from build123d import *

# Parameters (mm, degrees)
CROQUIS1_W              = 74
CROQUIS1_H              = 54
SALIENTE_EXTRUIR1_DEPTH = 6
CROQUIS3_W              = 9
CROQUIS3_H              = 5
SALIENTE_EXTRUIR2_DEPTH = 10
REDONDEO1_R             = 1
CORTAR_EXTRUIR1_DEPTH   = 100
CORTAR_EXTRUIR2_DEPTH   = 100
CORTAR_EXTRUIR3_DEPTH   = 70
CROQUIS8_W              = 8
CROQUIS8_H              = 6
CORTAR_EXTRUIR4_DEPTH   = 6
REDONDEO2_R             = 1
CROQUIS11_W             = 9
CROQUIS11_H             = 5
SALIENTE_EXTRUIR3_DEPTH = 5
REDONDEO3_R             = 1
CROQUIS17_R             = 1
CORTAR_EXTRUIR10_DEPTH  = 100
CROQUIS18_R             = 2
CORTAR_EXTRUIR11_DEPTH  = 1
CORTAR_EXTRUIR12_START  = -1
CROQUIS19_R             = 2
CORTAR_EXTRUIR12_DEPTH  = 1
CROQUIS12_R             = 1
CORTAR_EXTRUIR7_DEPTH   = 100
CROQUIS15_R             = 2
CORTAR_EXTRUIR8_DEPTH   = 1
CORTAR_EXTRUIR9_START   = -1
CROQUIS16_R             = 2
CORTAR_EXTRUIR9_DEPTH   = 1


with BuildPart() as part:
    # Croquis1 → Saliente-Extruir1 (new, symmetric)
    with BuildSketch(Plane(origin=(0, 0, 0), x_dir=(1, 0, 0), z_dir=(0, 1, 0))):
        Rectangle(CROQUIS1_W, CROQUIS1_H)
    extrude(amount=SALIENTE_EXTRUIR1_DEPTH, both=True)

    # Croquis3 → Saliente-Extruir2 (add, symmetric)
    with BuildSketch(Plane(origin=(0, 6, 0), x_dir=(1, 0, 0), z_dir=(0, 1, 0))):
        with Locations((0, -28.5)):
            Rectangle(CROQUIS3_W, CROQUIS3_H)
        with Locations((0, 28.5)):
            Rectangle(CROQUIS3_W, CROQUIS3_H)
    extrude(amount=SALIENTE_EXTRUIR2_DEPTH, both=True)

    # Redondeo1
    redondeo1_edges = [part.edges().sort_by_distance(p)[0] for p in [
        (4.5, 6, 31),
        (-4.5, 6, 31),
        (4.5, 6, -31),
        (-4.5, 6, -31),
    ]]
    fillet(redondeo1_edges, radius=REDONDEO1_R)

    # Croquis5 → Cortar-Extruir1 (cut)
    with BuildSketch(Plane(origin=(37, 0, 0), x_dir=(0, 0, -1), z_dir=(1, 0, 0))):
        with BuildLine():
            Line((-31, -1.820778385), (-31, -6))
            Line((-31, -6), (-18.642754783, -6))
            ThreePointArc((-18.642754783, -6), (-25.098766863, -4.730582529), (-31, -1.820778385))
        make_face()
        with BuildLine():
            Line((31, -1.820778385), (31, -6))
            Line((31, -6), (18.642754783, -6))
            ThreePointArc((18.642754783, -6), (25.098766863, -4.730582529), (31, -1.820778385))
        make_face()
    extrude(amount=-CORTAR_EXTRUIR1_DEPTH, mode=Mode.SUBTRACT)

    # Croquis6 → Cortar-Extruir2 (cut)
    with BuildSketch(Plane.ZY.offset(37)):
        with BuildLine():
            Line((-27, -1), (-27, -4))
            Line((-27, -4), (-31, -4))
            Line((-31, -4), (-33.432664366, -4))
            Line((-33.432664366, -4), (-33.432664366, 2.46409105))
            Line((-33.432664366, 2.46409105), (-31, 2.46409105))
            ThreePointArc((-31, 2.46409105), (-29.791283854, -0.181653154), (-27, -1))
        make_face()
        with BuildLine():
            Line((27, -1), (27, -4))
            Line((27, -4), (31, -4))
            Line((31, -4), (33.432664366, -4))
            Line((33.432664366, -4), (33.432664366, 2.46409105))
            Line((33.432664366, 2.46409105), (31, 2.46409105))
            ThreePointArc((31, 2.46409105), (29.791283854, -0.181653154), (27, -1))
        make_face()
    extrude(amount=-CORTAR_EXTRUIR2_DEPTH, mode=Mode.SUBTRACT)

    # Croquis7 → Cortar-Extruir3 (cut)
    with BuildSketch(Plane.ZY.offset(35)):
        with BuildLine():
            Line((-25, 6), (25, 6))
            Line((25, 6), (25, -2))
            ThreePointArc((25, -2), (21.888320303, -3.212786251), (18.642754783, -4))
            Line((18.642754783, -4), (-18.642754783, -4))
            ThreePointArc((-18.642754783, -4), (-21.888320303, -3.212786251), (-25, -2))
            Line((-25, -2), (-25, 6))
        make_face()
    extrude(amount=-CORTAR_EXTRUIR3_DEPTH, mode=Mode.SUBTRACT)

    # Croquis8 → Cortar-Extruir4 (cut)
    with BuildSketch(Plane.XZ.offset(6)):
        Polygon((-31.805445069, 16), (-28.194554931, 11.20818694), (-28.194554931, 13), (-21.194554931, 13), (-21.194554931, 19), (-28.194554931, 19), (-28.194554931, 20.79181306), align=None)
        Polygon((24.194554931, 13), (17.194554931, 13), (17.194554931, 19), (24.194554931, 19), (24.194554931, 20.79181306), (27.805445069, 16), (24.194554931, 11.20818694), align=None)
        with Locations((-2, 23)):
            Rectangle(CROQUIS8_W, CROQUIS8_H)
    extrude(amount=-CORTAR_EXTRUIR4_DEPTH, mode=Mode.SUBTRACT)

    # Redondeo2
    redondeo2_edges = [part.edges().sort_by_distance(p)[0] for p in [
        (-6, -4.802427791, 20),
        (2, -4.802427791, 20),
        (2, -2.203209257, 26),
        (-6, -2.203209257, 26),
    ]]
    fillet(redondeo2_edges, radius=REDONDEO2_R - 0.0001)  # a hair under: the kernel refuses the full size

    # Croquis11 → Saliente-Extruir3 (add, symmetric)
    with BuildSketch(Plane(origin=(0, 16, 0), x_dir=(1, 0, 0), z_dir=(0, 1, 0))):
        with Locations((0, -28.5)):
            Rectangle(CROQUIS11_W, CROQUIS11_H)
        with Locations((0, 28.5)):
            Rectangle(CROQUIS11_W, CROQUIS11_H)
    extrude(amount=SALIENTE_EXTRUIR3_DEPTH, both=True)

    # Redondeo3
    redondeo3_edges = [part.edges().sort_by_distance(p)[0] for p in [
        (-4.5, 16, -31),
        (4.5, 16, -31),
        (-4.5, 16, 31),
        (4.5, 16, 31),
    ]]
    fillet(redondeo3_edges, radius=REDONDEO3_R)

    # Croquis17 → Cortar-Extruir10 (cut)
    with BuildSketch(Plane.XY.offset(31)):
        with Locations((0, 18)):
            Circle(CROQUIS17_R)
    extrude(amount=-CORTAR_EXTRUIR10_DEPTH, mode=Mode.SUBTRACT)

    # Croquis18 → Cortar-Extruir11 (cut)
    with BuildSketch(Plane.XY.offset(31)):
        with Locations((0, 18)):
            Circle(CROQUIS18_R)
    extrude(amount=-CORTAR_EXTRUIR11_DEPTH, mode=Mode.SUBTRACT)

    # Croquis19 → Cortar-Extruir12 (cut)
    with BuildSketch(Plane(origin=(0, 0, -31), x_dir=(-1, 0, 0), z_dir=(0, 0, -1)).offset(CORTAR_EXTRUIR12_START)):
        with Locations(Location((0, 18, 0), (0, 0, 180))):
            Circle(CROQUIS19_R)
    extrude(amount=CORTAR_EXTRUIR12_DEPTH, mode=Mode.SUBTRACT)

    # Croquis12 → Cortar-Extruir7 (cut)
    with BuildSketch(Plane.XY.offset(31)):
        with Locations(Location((0, 18, 0), (0, 0, 180))):
            Circle(CROQUIS12_R)
    extrude(amount=-CORTAR_EXTRUIR7_DEPTH, mode=Mode.SUBTRACT)

    # Croquis15 → Cortar-Extruir8 (cut)
    with BuildSketch(Plane.XY.offset(31)):
        with Locations((0, 18)):
            Circle(CROQUIS15_R)
    extrude(amount=-CORTAR_EXTRUIR8_DEPTH, mode=Mode.SUBTRACT)

    # Croquis16 → Cortar-Extruir9 (cut)
    with BuildSketch(Plane(origin=(0, 0, -31), x_dir=(-1, 0, 0), z_dir=(0, 0, -1)).offset(CORTAR_EXTRUIR9_START)):
        with Locations(Location((0, 18, 0), (0, 0, 180))):
            Circle(CROQUIS16_R)
    extrude(amount=CORTAR_EXTRUIR9_DEPTH, mode=Mode.SUBTRACT)


solid = part.part
Source: CAD feature listing. Evaluate the final solid. Frame: model axes, mm. A direction names the side the tool comes from. Give positions to 0.01 mm unless a question says otherwise; leave off trailing zeros. Write each loop counter-clockwise with the first axis right and the second up, starting at its lowest first coordinate (ties: lowest second). Pieces come first, ordered by that corner, then holes. Notation, with made-up numbers: (18, 59.5) -> (63, 59.5) arc R32 cw to (63, 95.5) -> close; hole circle Ø5 at (-36.5, -5). An arc over 180 degrees is marked (long way). Return JSON: item names as keys, results as strings. Group by question number.
1. Mould query, pull axis Y, two halves, no side actions, for faces 5 (the face through (-25, -5, 19)), 6 (the face through (0.518, -5.376, -22.849)), 7 (the face through (-0.26, 16.017, -30.493)). Classes: +Y half, -Y half, draft (parallel to the pull), parting line (faces both ways), or undercut.
2. Pin query (flat end, axial travel): pin 1 Ø2 at (x, y) = (-1.5, -2.5) entering from -Z; pin 2 Ø18.5 at (x, z) = (-3, 7) entering from +Y; pin 3 Ø1.2 at (y, z) = (13.5, -27.5) entering from -X. Return the tip coordinate at first contact, or that it passes through.
3. Section B-B, the plane x = 22.5. Output: boundary loops of the cut face in (y, z).
4. Section C-C, the plane z = 23.5. Output: boundary loops of the cut face in (x, y), then the cut area to 3 significant figures.
5. Section D-D, the plane x = -15. Output: boundary loops of the cut face in (y, z), then the cut area to 3 significant figures.
6. Access query for faces 1 (the face through (1, 19, -30)), 2 (the face through (1, 17, 30)), 3 (the face through (0, 2, -25)), 4 (the face through (-21.195, -5, 16)). Directions: +Z, -Z, +X, -X, +Y, -Y. A direction counts if a zero-diameter tool reaches every point of the face in a straight line with its end or side. Return the directions, or none.
7. Material intervals for line 1 (Z direction, x = -12.5, y = -1.75); line 2 (X direction, y = 18, z = -26.8); line 3 (Y direction, x = 27.5, z = 0), sorted ascending. Write a range as from..to.
8. Section A-A, the plane y = 18. Output: boundary loops of the cut face in (x, z).
Determined:
{
 "1": {"face 5": "draft", "face 6": "-Y half", "face 7": "undercut"},
 "2": {"pin 1": "stops at z = -27", "pin 2": "stops at y = -4", "pin 3": "stops at x = -4.5"},
 "3": {"outline": "(-6, -18.64) arc R25 ccw to (-4, -27) -> (6, -27) -> (6, -25) -> (-2, -25) arc R25 cw to (-4, -18.64) -> (-4, 13) -> (-6, 13) -> close; (-5.98, 19) -> (-3.94, 19) arc R25 cw to (-2, 25) -> (6, 25) -> (6, 27) -> (-4, 27) arc R25 ccw to start"},
 "4": {"outline": "(-37, -5.21) -> (-6, -5.21) -> (-6, -2.64) -> (-35, -2.64) -> (-35, 6) -> (-37, 6) -> close; (2, -5.21) -> (37, -5.21) -> (37, 6) -> (35, 6) -> (35, -2.64) -> (2, -2.64) -> close", "area": "204 mm2"},
 "5": {"outline": "(-6, -18.64) arc R25 ccw to (-4, -27) -> (6, -27) -> (6, -25) -> (-2, -25) arc R25 cw to (-4, -18.64) -> (-4, 18.64) arc R25 cw to (-2, 25) -> (6, 25) -> (6, 27) -> (-4, 27) arc R25 ccw to (-6, 18.64) -> close", "area": "146 mm2"},
 "6": {"face 1": "-Z", "face 2": "+Z", "face 3": "+Y", "face 4": "+Y, -Y"},
 "7": {"line 1": "z = -27..-25, 25..27", "line 2": "x = -4.5..-1, 1..4.5", "line 3": "y = -6..-4"},
 "8": {"outline": "(-4.5, -30) arc R1 ccw to (-3.5, -31) -> (-2, -31) -> (-2, -30) -> (-1, -30) -> (-1, -26) -> (-4.5, -26) -> close; (-4.5, 26) -> (-1, 26) -> (-1, 30) -> (-2, 30) -> (-2, 31) -> (-3.5, 31) arc R1 ccw to (-4.5, 30) -> close; (1, -30) -> (2, -30) -> (2, -31) -> (3.5, -31) arc R1 ccw to (4.5, -30) -> (4.5, -26) -> (1, -26) -> close; (1, 26) -> (4.5, 26) -> (4.5, 30) arc R1 ccw to (3.5, 31) -> (2, 31) -> (2, 30) -> (1, 30) -> close"}
}
